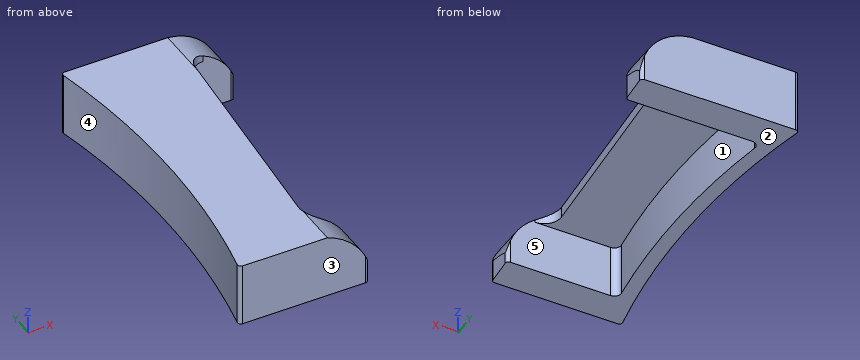
```python
from build123d import *

# Parameters (mm, degrees)
F1_DEPTH = 24.384
F3_DEPTH = 20.32
F6_DEPTH = 124.001
F7_DEPTH = 19.5072


with BuildPart() as f1:
    # F0 (on Top) → F1 (new body)
    with BuildSketch(Plane.XY):
        with BuildLine():
            Line((59.612351, 0), (1.573374, 0))
            ThreePointArc((1.573374, 0), (0.586221, -0.470982), (0.331244, -1.5346))
            ThreePointArc((0.331244, -1.5346), (6.7, -62), (0.331244, -122.4654))
            ThreePointArc((0.331244, -122.4654), (0.586221, -123.529018), (1.573374, -124))
            Line((1.573374, -124), (48.837674, -124))
            ThreePointArc((48.837674, -124), (49.695106, -123.666862), (50.102706, -122.842221))
            Line((50.102706, -122.842221), (51.003997, -112.682221))
            ThreePointArc((51.003997, -112.682221), (50.675826, -111.712568), (49.738964, -111.3))
            Line((49.738964, -111.3), (40.215034, -111.3))
            ThreePointArc((40.215034, -111.3), (35.530725, -109.237161), (33.889873, -104.388897))
            Line((33.889873, -104.388897), (41.510034, -18.488897))
            ThreePointArc((41.510034, -18.488897), (43.548034, -14.365691), (47.835195, -12.7))
            Line((47.835195, -12.7), (58.711061, -12.7))
            ThreePointArc((58.711061, -12.7), (59.568493, -12.366862), (59.976093, -11.542221))
            Line((59.976093, -11.542221), (60.877384, -1.382221))
            ThreePointArc((60.877384, -1.382221), (60.549213, -0.412568), (59.612351, 0))
        make_face()
    extrude(amount=F1_DEPTH)

    # F2 (on face) → F3 (cut)
    with BuildSketch(Plane(origin=(0, 0, 0), x_dir=(1, 0, 0), z_dir=(0, 0, -1))):
        with BuildLine():
            ThreePointArc((11.140821, 111.3), (9.209142, 110.409307), (8.632213, 108.361901))
            ThreePointArc((8.632213, 108.361901), (12.288, 62), (8.632213, 15.638099))
            ThreePointArc((8.632213, 15.638099), (9.209142, 13.590693), (11.140821, 12.7))
            Line((11.140821, 12.7), (59.612351, 12.7))
            Line((59.612351, 12.7), (48.837674, 111.3))
            Line((48.837674, 111.3), (11.140821, 111.3))
        make_face()
    extrude(amount=-F3_DEPTH, mode=Mode.SUBTRACT)

    # F4 (on face) → F6 (cut, through all)
    with BuildSketch(Plane(origin=(0, 0, 0), x_dir=(-1, 0, 0), z_dir=(0, 1, 0))):
        with BuildLine():
            Line((-60.905915, 0), (-60.905915, 1.609697))
            ThreePointArc((-60.905915, 1.609697), (-55.623214, 16.900361), (-41.280743, 24.384))
            Line((-41.280743, 24.384), (-40.572539, 44.529654))
            Line((-40.572539, 44.529654), (-74.00889, 45.705081))
            Line((-74.00889, 45.705081), (-79.637952, 1.058017))
            Line((-79.637952, 1.058017), (-60.905915, 0))
        make_face()
    extrude(amount=-F6_DEPTH, mode=Mode.SUBTRACT)

    # F5 (on face) → F7 (cut)
    with BuildSketch(Plane.XZ.offset(124)):
        with BuildLine():
            ThreePointArc((34.204833, 24.384), (46.666601, 14.917599), (51.396679, 0))
            Line((51.396679, 0), (51.396679, 24.384))
            Line((51.396679, 24.384), (34.204833, 24.384))
        make_face()
    extrude(amount=-F7_DEPTH, mode=Mode.SUBTRACT)


solid = f1.part
```
Source: CAD feature listing. Evaluate the final solid. Frame: model axes, mm. Face numbers are marked on the shaded views. A direction names the side the tool comes from. Round coordinates to 2 decimals unless told otherwise and drop trailing zeros. Loops run counter-clockwise (first coordinate to the right, second up) from the corner with the lowest first, then second, coordinate; pieces in that order, holes last.
1. Contact query for flat-ended pins moving along their axis: pin 1 (4 mm diameter, centred on x = 33.5, y = -27, fed in from -Z); pin 2 (8 mm diameter, centred on y = -110, z = 6, fed in from +X); pin 3 (5 mm diameter, centred on y = -84, z = 17, fed in from +X). Output: stop coordinate, or through.
2. Mould query, pull axis Y, two halves, no side actions, for the marked faces 1, 2 and 3. Classes: released by +Y, released by -Y, zero draft, split by the parting line, or undercut.
3. Section query B-B on x = 29.5. Output: boundary loops of the cut face in (y, z).
4. Ray query, L1, parallel to Y at x = 21.5, z = 5.5; L2, parallel to X at y = -64.5, z = 9; L3, parallel to Z at x = 11, y = -31. Return the intervals inside material, ascending.
5. Access query for the marked faces 4 and 5. Directions: +Z, -Z, +X, -X, +Y, -Y. A direction counts if a zero-diameter tool reaches every point of the face in a straight line with its end or side. Return the directions, or none.
6. Section query A-A on z = 2.25. Output: boundary loops of the cut face in (x, y).
7. Section query C-C on y = -85. Output: boundary loops of the cut face in (x, z), and give its area (3 significant figures).
8. Section query D-D on z = 18.5. Output: boundary loops of the cut face in (x, y), and give its area (3 significant figures).
Answers below:
1. pin 1: stops at z = 20.32
1. pin 2: stops at x = 51.01
1. pin 3: stops at x = 11.64
2. face 1: undercut
2. face 2: zero draft
2. face 3: released by -Y
3. outline: (-124, 0) - (-111.3, 0) - (-111.3, 20.32) - (-12.7, 20.32) - (-12.7, 0) - (0, 0) - (0, 24.38) - (-124, 24.38) - close
4. L1: y = -124 to -111.3, -12.7 to 0
4. L2: x = 6.69 to 12.28
4. L3: z = 20.32 to 24.38
5. face 4: +Z, -Z, -X
5. face 5: -Z, +X
6. outline: (0.33, -122.47) arc R1.27 ccw to (1.57, -124) - (48.84, -124) arc R1.27 ccw to (50.1, -122.84) - (51, -112.68) arc R1.27 ccw to (49.74, -111.3) - (11.14, -111.3) arc R2.54 cw to (8.63, -108.36) arc R295.8 ccw to (8.63, -15.64) arc R2.54 cw to (11.14, -12.7) - (58.71, -12.7) arc R1.27 ccw to (59.98, -11.54) - (60.88, -1.38) arc R1.27 ccw to (59.61, 0) - (1.57, 0) arc R1.27 ccw to (0.33, -1.53) arc R290.22 cw to start
7. outline: (5.79, 0) - (11.39, 0) - (11.39, 20.32) - (35.61, 20.32) - (35.61, 24.38) - (5.79, 24.38) - close
7. area: 235 mm2
8. outline: (0.33, -122.47) arc R1.27 ccw to (1.57, -124) - (43.62, -124) - (43.62, -111.3) - (11.14, -111.3) arc R2.54 cw to (8.63, -108.36) arc R295.8 ccw to (8.63, -15.64) arc R2.54 cw to (11.14, -12.7) - (54.1, -12.7) - (54.1, 0) - (1.57, 0) arc R1.27 ccw to (0.33, -1.53) arc R290.22 cw to start
8. area: 1,760 mm2
